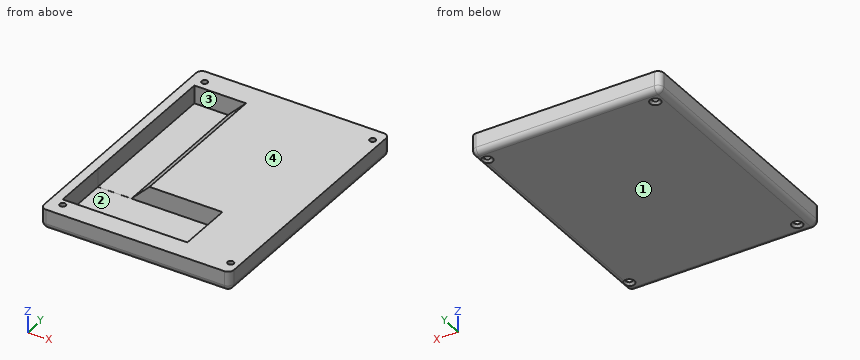
```python
from build123d import *

# Parameters (mm, degrees)
SKETCH060_W     = 81.930373
SKETCH060_H     = 8.636624
PAD014_DEPTH    = 109
FILLET032_R     = 2.5
SKETCH061_W     = 53.822303
SKETCH061_H     = 19.035354
POCKET028_DEPTH = 24
SKETCH062_W     = 14.825619
SKETCH062_H     = 9.085716
POCKET029_DEPTH = 66
CHAMFER015_SIZE = 7.5
SKETCH063_R     = 1.3
POCKET030_DEPTH = 8.637624
CHAMFER016_SIZE = 1


with BuildPart() as part:
    # Sketch060 → Pad014 (new body)
    with BuildSketch(Plane.XZ.offset(-61)):
        with Locations((-3.438551, -16.819782)):
            Rectangle(SKETCH060_W, SKETCH060_H)
    extrude(amount=PAD014_DEPTH)

    # Fillet032
    fillet032_edges = [part.edges().sort_by_distance(p)[0] for p in [
        (-44.403737, 61, -16.819782),
        (37.526636, 61, -16.819782),
        (-3.43855, 61, -21.138094),
        (-44.403737, 6.5, -21.138094),
        (37.526636, 6.5, -21.138094),
        (37.526636, -48, -16.819782),
        (-3.43855, -48, -21.138094),
        (-44.403737, -48, -16.819782),
    ]]
    fillet(fillet032_edges, radius=FILLET032_R)

    # Sketch061 → Pocket028 (cut)
    with BuildSketch(Plane.XZ.offset(39)):
        with Locations((-13.565516, -10.812245)):
            Rectangle(SKETCH061_W, SKETCH061_H)
    extrude(amount=-POCKET028_DEPTH, mode=Mode.SUBTRACT)

    # Sketch062 → Pocket029 (cut)
    with BuildSketch(Plane.XZ.offset(15)):
        with Locations((-33.055162, -15.752031)):
            Rectangle(SKETCH062_W, SKETCH062_H)
    extrude(amount=-POCKET029_DEPTH, mode=Mode.SUBTRACT)

    # Chamfer015
    chamfer015_edges = [part.edges().sort_by_distance(p)[0] for p in [
        (-25.642353, 18, -12.50147),
    ]]
    chamfer(chamfer015_edges, length=CHAMFER015_SIZE)

    # Sketch063 (on Face28 of Chamfer015) → Pocket030 (cut, through all)
    with BuildSketch(Plane(origin=(0, 0, -21.138094), x_dir=(1, 0, 0), z_dir=(0, 0, -1))):
        with Locations((-38.519981, 42.037067)):
            Circle(SKETCH063_R)
        with Locations((34.008266, 42.037067)):
            Circle(SKETCH063_R)
        with Locations((34.008266, -54.977215)):
            Circle(SKETCH063_R)
        with Locations((-38.519981, -54.977215)):
            Circle(SKETCH063_R)
    extrude(amount=-POCKET030_DEPTH, mode=Mode.SUBTRACT)

    # Chamfer016
    chamfer016_edges = [part.edges().sort_by_distance(p)[0] for p in [
        (32.708266, -42.037067, -21.138094),
        (32.708266, 54.977215, -21.138094),
        (-39.819981, 54.977215, -21.138094),
        (-39.819981, -42.037067, -21.138094),
    ]]
    chamfer(chamfer016_edges, length=CHAMFER016_SIZE)


solid = part.part
```
Here's how the part is built. I have some questions about the finished solid (model axes, mm). Face numbers are marked on the shaded views. A direction names the side the tool comes from. Coordinates: 2 decimals unless noted, no trailing zeros. Order: outer loops, then holes, each group sorted by start corner. A loop starts at its lowest first (then second) coordinate and runs counter-clockwise, first axis right, second up. Notation, with made-up numbers: (-19.75, -36) -> (31.25, -36) arc R20 cw to (31.25, 0) -> close; hole circle Ø6 at (75, 21.5). An arc over 180 degrees is marked (long way). Return JSON: item names as keys, results as strings.
1) I'm going to push flat-ended pins straight in: P1, Ø2, axis at y = 25, z = -19, coming from the -X side; P2, Ø3.5, axis at x = 34.01, y = 54.98, coming from the -Z side; P3, Ø12, axis at x = -31, y = 19.5, coming from the +Z side. Where does each tip first touch, or does it pass through?
Conclusion:
{"P1": "stops at x = -44.4", "P2": "stops at z = -20.59", "P3": "stops at z = -19.36"}
2) If I drill on probe 1 along Y at (x, z) = (-12.5, -15); probe 2 along Y at (x, z) = (34, -13.25); probe 3 along Y at (x, z) = (-34.5, -14.75), over which ranges is the centre line in solid material (lowest first)?
Conclusion:
{"probe 1": "y = -48 to -39, -15 to 61", "probe 2": "y = -48 to -43.34, -40.74 to 53.68, 56.28 to 61", "probe 3": "y = -48 to -39, 51 to 61"}
3) If we section it at C-C on z = -16.5: State how many separate pieces and enclosed holes the cut face has, plus the area to 3 significant figures.
Conclusion:
{"separate pieces": "1", "enclosed holes": "5", "area": "6,400 mm²"}
4) Thinking about a two-plate mould opening in Y: for the marked faces 1 and 2, which applies, +Y half, -Y half, draft (parallel to the pull), parting line (faces both ways), or undercut?
Conclusion:
{"face 1": "draft", "face 2": "undercut"}
5) If we section it at B-B on x = -17: List the corners of the cut face in (y, z) for me.
Conclusion:
{"outline": "(-48, -18.64) arc R2.5 ccw to (-45.5, -21.14) -> (58.5, -21.14) arc R2.5 ccw to (61, -18.64) -> (61, -12.5) -> (-15, -12.5) -> (-15, -20.33) -> (-39, -20.33) -> (-39, -12.5) -> (-48, -12.5) -> close"}
6) On a 3-axis mill with a long thin cutter (end or side, diameter ignored), from which of +Z, -Z, +X, -X, +Y, -Y can I reach the whole of each face in a straight line? I mean the marked faces 3 and 4. Say none if no direction works.
Conclusion:
{"face 3": "+Z", "face 4": "+Z, +X, -X, +Y, -Y"}
7) If we section it at A-A on y = -19.5: List the corners of the cut face in (x, z) for me.
Conclusion:
{"outline": "(-44.4, -18.64) arc R2.5 ccw to (-41.9, -21.14) -> (35.03, -21.14) arc R2.5 ccw to (37.53, -18.64) -> (37.53, -12.5) -> (13.35, -12.5) -> (13.35, -20.33) -> (-40.48, -20.33) -> (-40.48, -12.5) -> (-44.4, -12.5) -> close"}
